from build123d import *

# Parameters (mm, degrees)
SKETCH1_W           = 90.17
SKETCH1_H           = 90.17
BOSS_EXTRUDE1_DEPTH = 34.163
CUT_EXTRUDE1_DEPTH  = 91.17
SKETCH3_W           = 78.994
SKETCH3_H           = 42.418
CUT_EXTRUDE2_DEPTH  = 0.762
SKETCH4_W           = 79.7814
SKETCH4_H           = 9.398
SKETCH4_W_2         = 77.7494
SKETCH4_H_2         = 7.366
BOSS_EXTRUDE2_DEPTH = 0.762
SKETCH5_R           = 1.905
CUT_EXTRUDE3_DEPTH  = 5.08
FILLET1_R           = 0.508


with BuildPart() as part:
    # Sketch1 → Boss-Extrude1 (new body)
    with BuildSketch(Plane(origin=(0, 0, 0), x_dir=(1, 0, 0), z_dir=(0, 1, 0))):
        Rectangle(SKETCH1_W, SKETCH1_H)
    extrude(amount=BOSS_EXTRUDE1_DEPTH)

    # Sketch2 → Cut-Extrude1 (cut, through all)
    with BuildSketch(Plane(origin=(45.085, 0, 0), x_dir=(0, 0, -1), z_dir=(1, 0, 0))):
        Polygon((-45.085, 24.13), (-45.085, 34.163), (-22.86, 34.163), (-31.877, 24.13), align=None)
        Polygon((45.085, 24.13), (45.085, 34.163), (22.86, 34.163), (31.877, 24.13), align=None)
    extrude(amount=-CUT_EXTRUDE1_DEPTH, mode=Mode.SUBTRACT)

    # Sketch3 → Cut-Extrude2 (cut)
    with BuildSketch(Plane(origin=(0, 34.163, 0), x_dir=(1, 0, 0), z_dir=(0, 1, 0))):
        Rectangle(SKETCH3_W, SKETCH3_H)
    extrude(amount=-CUT_EXTRUDE2_DEPTH, mode=Mode.SUBTRACT)

    # Sketch4 → Boss-Extrude2 (add)
    with BuildSketch(Plane(origin=(0, 24.13, 0), x_dir=(1, 0, 0), z_dir=(0, 1, 0))):
        with Locations((0, 38.481)):
            Rectangle(SKETCH4_W, SKETCH4_H)
        with Locations((0, 38.481)):
            Rectangle(SKETCH4_W_2, SKETCH4_H_2, mode=Mode.SUBTRACT)
    boss_extrude2 = extrude(amount=BOSS_EXTRUDE2_DEPTH)

    # Sketch5 → Cut-Extrude3 (cut)
    with BuildSketch(Plane(origin=(0, 24.13, 0), x_dir=(1, 0, 0), z_dir=(0, 1, 0))):
        with Locations((-2.54, 38.481)):
            Circle(SKETCH5_R)
        with Locations((-7.62, 38.481)):
            Circle(SKETCH5_R)
        with Locations((-12.7, 38.481)):
            Circle(SKETCH5_R)
        with Locations((-17.78, 38.481)):
            Circle(SKETCH5_R)
        with Locations((-22.86, 38.481)):
            Circle(SKETCH5_R)
        with Locations((-27.94, 38.481)):
            Circle(SKETCH5_R)
        with Locations((27.94, 38.481)):
            Circle(SKETCH5_R)
        with Locations((22.86, 38.481)):
            Circle(SKETCH5_R)
        with Locations((17.78, 38.481)):
            Circle(SKETCH5_R)
        with Locations((12.7, 38.481)):
            Circle(SKETCH5_R)
        with Locations((7.62, 38.481)):
            Circle(SKETCH5_R)
        with Locations((2.54, 38.481)):
            Circle(SKETCH5_R)
    cut_extrude3 = extrude(amount=-CUT_EXTRUDE3_DEPTH, mode=Mode.SUBTRACT)

    # Mirror1: Boss-Extrude2, Cut-Extrude3 across plane
    add(boss_extrude2.mirror(Plane.XY))
    add(cut_extrude3.mirror(Plane.XY), mode=Mode.SUBTRACT)

    # Fillet1
    fillet1_edges = [part.edges().sort_by_distance(p)[0] for p in [
        (45.085, 34.163, 0),
        (-45.085, 34.163, 0),
        (45.085, 12.065, 45.085),
        (-45.085, 12.065, 45.085),
        (-45.085, 12.065, -45.085),
        (45.085, 12.065, -45.085),
        (-45.085, 24.13, 38.481),
        (0, 24.13, 31.877),
        (0, 24.13, 45.085),
        (-45.085, 29.1465, 27.3685),
        (0, 34.163, 22.86),
        (45.085, 24.13, 38.481),
        (45.085, 29.1465, 27.3685),
        (-45.085, 24.13, -38.481),
        (0, 24.13, -45.085),
        (-45.085, 29.1465, -27.3685),
        (0, 24.13, -31.877),
        (0, 34.163, -22.86),
        (45.085, 24.13, -38.481),
        (45.085, 29.1465, -27.3685),
        (39.497, 34.163, 0),
        (0, 34.163, -21.209),
        (-39.497, 34.163, 0),
        (0, 34.163, 21.209),
        (0, 0, 45.085),
        (-45.085, 0, 0),
        (0, 0, -45.085),
        (45.085, 0, 0),
    ]]
    fillet(fillet1_edges, radius=FILLET1_R)


solid = part.part
Geometry: final body of the model. Coordinates: model frame, mm. A direction names the side the tool comes from. Give positions to 0.01 mm unless a question says otherwise; leave off trailing zeros. Order: outer loops, then holes, each group sorted by start corner. A loop starts at its lowest first (then second) coordinate and runs counter-clockwise, first axis right, second up. Notation, with made-up numbers: (-8.75, 52.5) -> (27.25, 52.5) arc R26 cw to (27.25, 82.5) -> close; hole circle Ø6 at (57, 28). An arc over 180 degrees is marked (long way). Write each question's results on one line, items separated by ' | '.
1) Draft query along X for faces 1 (the face through (-3, 24.13, -33)), 2 (the face through (-44.94, 29.112, -27.194)), 3 (the face through (-16.9, 21.63, -36.79)). Return one class per face: released by +X, released by -X, zero draft, split by the parting line, or undercut.
Geometry says:
face 1: zero draft | face 2: released by -X | face 3: undercut
2) First-contact query: pin 1 Ø0.6 at (y, z) = (24.5, -38) entering from -X; pin 2 Ø1.1 at (x, z) = (2.5, -38) entering from +Y; pin 3 Ø2 at (x, z) = (-24, 8.5) entering from +Y; pin 4 Ø4.5 at (x, z) = (12.7, -38.481) entering from -Y. Flat tips, straight axial feed; report the tip coordinate or a pass-through.
Geometry says:
pin 1: stops at x = -39.89 | pin 2: stops at y = 19.05 | pin 3: stops at y = 33.4 | pin 4: stops at y = 0
3) Cut plane A-A (z = -19). Output: boundary loops of the cut face in (x, y) (3 decimals).
Geometry says:
outline: (-45.085, 0.508) arc R0.508 ccw to (-44.577, 0) -> (44.577, 0) arc R0.508 ccw to (45.085, 0.508) -> (45.085, 33.655) arc R0.508 ccw to (44.577, 34.163) -> (40.005, 34.163) arc R0.508 ccw to (39.497, 33.655) -> (39.497, 33.401) -> (-39.497, 33.401) -> (-39.497, 33.655) arc R0.508 ccw to (-40.005, 34.163) -> (-44.577, 34.163) arc R0.508 ccw to (-45.085, 33.655) -> close
4) Line query: line 1 along Z through (x, y) = (22.86, 20.25) (3 decimals); line 2 along Z through (x, y) = (12, 22) (3 decimals); line 3 along Y through (x, z) = (-7.5, 15.5). Output: solid intervals per line, ascending.
Geometry says:
line 1: z = -45.085 to -40.386, -36.576 to 36.576, 40.386 to 45.085 | line 2: z = -45.085 to -40.253, -36.709 to 36.709, 40.253 to 45.085 | line 3: y = 0 to 33.4
5) Set-up query: faces 4 (the face through (0, 34.163, -22)), 5 (the face through (8, 19.05, 39)). Return all of +Z, -Z, +X, -X, +Y, -Y with unobstructed straight access to the full face (end or side cutting, diameter ignored); none if empty.
Geometry says:
face 4: +Z, -Z, +X, -X, +Y | face 5: +Y
